```python
from build123d import *

# Parameters (mm, degrees)
BOSS_EXTRUDE1_DEPTH      = 2.5
BOSS_EXTRUDE1_DEPTH_BACK = 2.5
SKETCH1_R                = 2.13
SKETCH2_R                = 2.55
BOSS_EXTRUDE2_DEPTH      = 4


with BuildPart() as part:
    # Sketch1 → Boss-Extrude1 (new, two sides: drawn at the far end of the back side and taken through both)
    with BuildSketch(Plane(origin=(0, 0, 0), x_dir=(1, 0, 0), z_dir=(0, 1, 0)).offset(-BOSS_EXTRUDE1_DEPTH_BACK)):
        with BuildLine():
            Line((-13.675, 3.75), (13.675, 3.75))
            ThreePointArc((13.675, 3.75), (17.425, 0), (13.675, -3.75))
            Line((13.675, -3.75), (-13.675, -3.75))
            ThreePointArc((-13.675, -3.75), (-17.425, 0), (-13.675, 3.75))
        make_face()
        with Locations(Location((0, 0, 0), (0, 0, 270))):
            Circle(SKETCH1_R, mode=Mode.SUBTRACT)
    extrude(amount=BOSS_EXTRUDE1_DEPTH + BOSS_EXTRUDE1_DEPTH_BACK)

    # Sketch2 → Boss-Extrude2 (add)
    with BuildSketch(Plane(origin=(0, 2.5, 0), x_dir=(1, 0, 0), z_dir=(0, 1, 0))):
        with Locations(Location((-13.675, 0, 0), (0, 0, 270))):
            Circle(SKETCH2_R)
        with Locations(Location((13.675, 0, 0), (0, 0, 270))):
            Circle(SKETCH2_R)
    extrude(amount=BOSS_EXTRUDE2_DEPTH)


solid = part.part
```
For this review, take the finished solid that the model builds, in its own axes (mm). A direction names the side the tool comes from. Coordinates: 2 decimals unless noted, no trailing zeros. Write each loop counter-clockwise with the first axis right and the second up, starting at its lowest first coordinate (ties: lowest second). Pieces come first, ordered by that corner, then holes.
(1) The part is to be moulded in two halves that separate along Z. For faces 3 (the face through (0, 0, 3.75)), 4 (the face through (0, -2.5, -3)), 5 (the face through (-1.296, -0.035, -1.69)), say which applies: +Z half, -Z half, draft (parallel to the pull), parting line (faces both ways), or undercut.
(2) Add section C-C on z = -1.75. Give the boundary of the cut face in (x, y).
(3) Add section B-B on x = 0. Give the boundary of the cut face in (y, z).
(4) Wall thickness on probe 1 along X at (y, z) = (0, 0) (3 decimals); probe 2 along Y at (x, z) = (-8.5, -1.75); probe 3 along X at (y, z) = (5.75, 2.25) (3 decimals): over which ranges is each line inside the solid? List them lowest first.
(5) For pin 1 Ø1 at (x, y) = (11.5, 4.5) entering from +Z; pin 2 Ø4 at (x, z) = (-11, -3) entering from +Y; pin 3 Ø2 at (x, z) = (3.5, 0.5) entering from +Y; pin 4 Ø4 at (y, z) = (5, -1) entering from -X (3 decimals), all flat-tipped, find the tip position at first contact; note any pin that passes through.
(6) Tool access review of faces 1 (the face through (14, 6.5, 0)), 2 (the face through (-11.147, 4.472, -0.332)): name each direction out of +Z, -Z, +X, -X, +Y, -Y from which nothing blocks a thin tool from reaching the whole face with its end or side.
(7) Add section A-A on z = 0. Give the boundary of the cut face in (x, y) (3 decimals).
(8) Add section D-D on x = 6. Give the boundary of the cut face in (y, z), then the cut area to 3 significant figures.
Answer sheet:
1. face 3: +Z half
1. face 4: draft
1. face 5: undercut
2. outline: (-16.99, -2.5) - (-1.21, -2.5) - (-1.21, 2.5) - (-11.82, 2.5) - (-11.82, 6.5) - (-15.53, 6.5) - (-15.53, 2.5) - (-16.99, 2.5) - close; (1.21, -2.5) - (16.99, -2.5) - (16.99, 2.5) - (15.53, 2.5) - (15.53, 6.5) - (11.82, 6.5) - (11.82, 2.5) - (1.21, 2.5) - close
3. outline: (-2.5, -3.75) - (2.5, -3.75) - (2.5, -2.13) - (-2.5, -2.13) - close; (-2.5, 2.13) - (2.5, 2.13) - (2.5, 3.75) - (-2.5, 3.75) - close
4. probe 1: x = -17.425 to -2.13, 2.13 to 17.425
4. probe 2: y = -2.5 to 2.5
4. probe 3: x = -14.875 to -12.475, 12.475 to 14.875
5. pin 1: stops at z = 1.92
5. pin 2: stops at y = 6.5
5. pin 3: stops at y = 2.5
5. pin 4: stops at x = -16.225
6. face 1: +Z, -Z, +X, -X, +Y
6. face 2: +Y
7. outline: (-17.425, -2.5) - (-2.13, -2.5) - (-2.13, 2.5) - (-11.125, 2.5) - (-11.125, 6.5) - (-16.225, 6.5) - (-16.225, 2.5) - (-17.425, 2.5) - close; (2.13, -2.5) - (17.425, -2.5) - (17.425, 2.5) - (16.225, 2.5) - (16.225, 6.5) - (11.125, 6.5) - (11.125, 2.5) - (2.13, 2.5) - close
8. outline: (-2.5, -3.75) - (2.5, -3.75) - (2.5, 3.75) - (-2.5, 3.75) - close
8. area: 37.5 mm2
